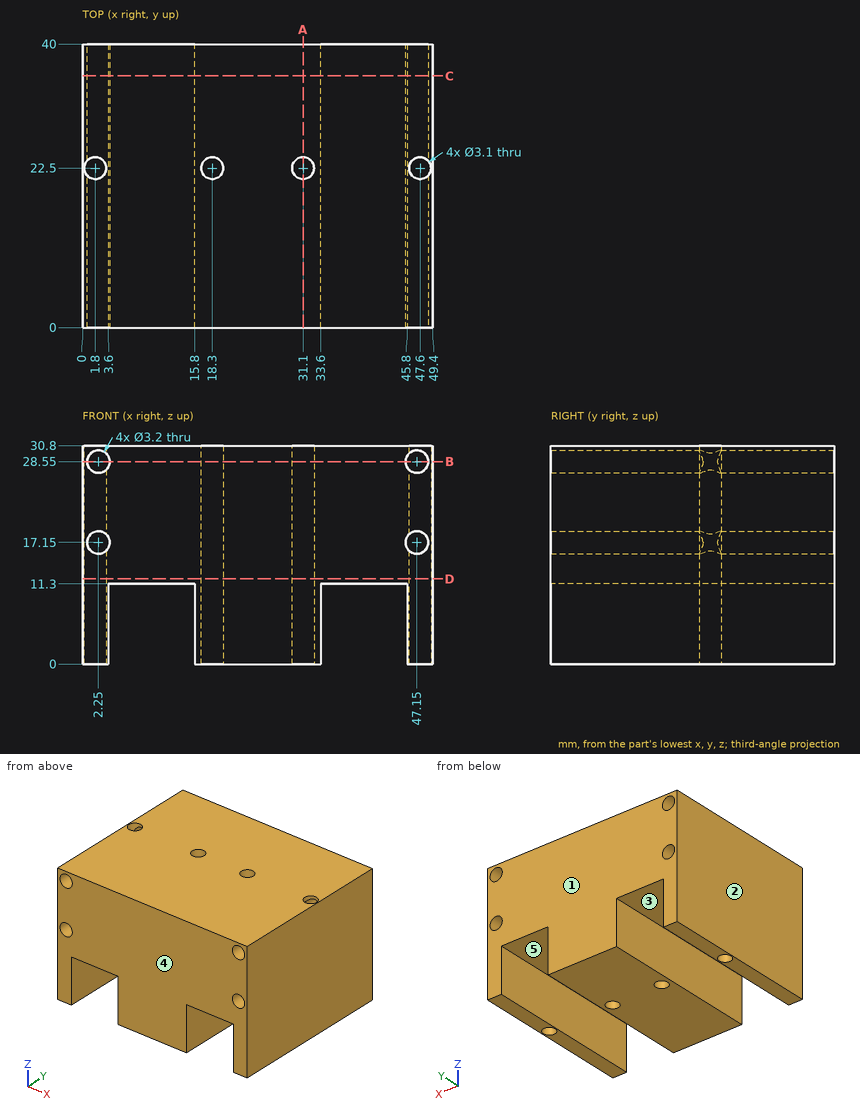
Job drawing, mm, ordinate dimensions from the low corner. One solid piece. A direction names the side the tool comes from. Round coordinates to 2 decimals unless told otherwise and drop trailing zeros. Loops run counter-clockwise (first coordinate to the right, second up) from the corner with the lowest first, then second, coordinate; pieces in that order, holes last.
Item 1: Cut at B-B, the plane z = 28.55. Give the cut face in (x, y).
Item 2: Drop a flat-ended pin along its axis: P1, Ø3, axis at x = 18.3, y = 22.5, coming from the -Z side. Give the stop position or say it passes through.
Item 3: Cut at C-C, the plane y = 35.5. Give the cut face in (x, z), then the cut area to 3 significant figures.
Item 4: Cut at D-D, the plane z = 12. Give the cut face in (x, y).
Item 5: Drill centre lines: line 1 (X direction, y = 26, z = 4); line 2 (X direction, y = 16, z = 28); line 3 (Z direction, x = 9.5, y = 32). Where is each one in solid material? Low to high.
Item 6: Mould opens along X. For the marked faces 1, 2 and 3 say: +X half, -X half, draft (parallel to the pull), parting line (faces both ways), or undercut.
Item 7: Cut at A-A, the plane x = 31.1. Give the cut face in (y, z).
Item 8: 3-axis set-ups, long thin cutter, end or side, ignore diameter. For the marked faces 4 and 5: which of +Z, -Z, +X, -X, +Y, -Y reach the whole face in a straight line?
A:
1. outline: (0, 0) - (0.65, 0) - (0.65, 21.46) arc R1.55 cw to (0.65, 23.54) - (0.65, 40) - (0, 40) - close; (3.85, 0) - (45.55, 0) - (45.55, 40) - (3.85, 40) - close; (48.75, 0) - (49.4, 0) - (49.4, 40) - (48.75, 40) - (48.75, 23.54) arc R1.55 cw to (48.75, 21.46) - close; hole circle Ø3.1 at (18.3, 22.5); hole circle Ø3.1 at (31.1, 22.5)
2. P1: passes through
3. outline: (0, 0) - (3.6, 0) - (3.6, 11.3) - (15.8, 11.3) - (15.8, 0) - (33.6, 0) - (33.6, 11.3) - (45.8, 11.3) - (45.8, 0) - (49.4, 0) - (49.4, 30.8) - (0, 30.8) - close; hole circle Ø3.2 at (2.25, 17.15); hole circle Ø3.2 at (2.25, 28.55); hole circle Ø3.2 at (47.15, 17.15); hole circle Ø3.2 at (47.15, 28.55)
3. area: 1,210 mm2
4. outline: (0, 0) - (49.4, 0) - (49.4, 40) - (0, 40) - close; hole circle Ø3.1 at (1.8, 22.5); hole circle Ø3.1 at (18.3, 22.5); hole circle Ø3.1 at (31.1, 22.5); hole circle Ø3.1 at (47.6, 22.5)
5. line 1: x = 0 to 3.6, 15.8 to 33.6, 45.8 to 49.4
5. line 2: x = 0 to 0.75, 3.75 to 45.65, 48.65 to 49.4
5. line 3: z = 11.3 to 30.8
6. face 1: draft
6. face 2: -X half
6. face 3: undercut
7. outline: (0, 0) - (20.95, 0) - (20.95, 30.8) - (0, 30.8) - close; (24.05, 0) - (40, 0) - (40, 30.8) - (24.05, 30.8) - close
8. face 4: +Z, -Z, +X, -X, -Y
8. face 5: -Z, +Y, -Y
